```python
from build123d import *

# Parameters (mm, degrees)
F1_W     = 30
F1_H     = 30
F1_W_2   = 27
F1_H_2   = 27
F3_R     = 5
F5_DEPTH = 40
F4_R     = 5
F6_DEPTH = 40


with BuildPart() as f2:
    # F2: sweep along a path in F0
    with BuildLine(Plane.YZ) as f2_path:
        Line((0, 0), (0, 750))
        ThreePointArc((0, 750), (29.2893218813, 820.7106781187), (100, 850))
        Line((100, 850), (368.5786437627, 850))
        ThreePointArc((368.5786437627, 850), (406.8469869992, 842.3879532511), (439.2893218813, 820.7106781187))
        Line((439.2893218813, 820.7106781187), (470.7106781187, 789.2893218813))
        ThreePointArc((470.7106781187, 789.2893218813), (503.1530130008, 767.6120467489), (541.4213562373, 760))
        Line((541.4213562373, 760), (820, 760))
        ThreePointArc((820, 760), (890.7106781187, 730.7106781187), (920, 660))
        Line((920, 660), (920, 0))
    # F1 (on Top) → F2 (sweep)
    with BuildSketch(Plane.XY):
        Rectangle(F1_W, F1_H)
        Rectangle(F1_W_2, F1_H_2, mode=Mode.SUBTRACT)
    sweep(path=f2_path.line)

    # F3 (on face) → F5 (cut)
    with BuildSketch(Plane.XY.offset(865)):
        with Locations((0, 130)):
            Circle(F3_R)
        with Locations((0, 338.5786437627)):
            Circle(F3_R)
    extrude(amount=-F5_DEPTH, mode=Mode.SUBTRACT)

    # F4 (on face) → F6 (cut)
    with BuildSketch(Plane.XY.offset(775)):
        with Locations((0, 571.4213562373)):
            Circle(F4_R)
        with Locations((0, 790)):
            Circle(F4_R)
    extrude(amount=-F6_DEPTH, mode=Mode.SUBTRACT)


solid = f2.part
```
Geometry: final body of the model. Coordinates: model frame, mm. A direction names the side the tool comes from. Coordinates: 2 decimals unless noted, no trailing zeros. Order: outer loops, then holes, each group sorted by start corner. A loop starts at its lowest first (then second) coordinate and runs counter-clockwise, first axis right, second up. Notation, with made-up numbers: (-1, 42.25) -> (28, 42.25) arc R32 ccw to (28, 81.25) -> close; hole circle Ø11 at (83, -14.75). An arc over 180 degrees is marked (long way). Write each question's results on one line, items separated by ' | '. Start each with the question number.
1) Cut plane C-C, the plane x = 0. State how many separate pieces and enclosed holes the cut face has, and give its area (3 significant figures).
2) First-contact query: pin 1 (15 mm diameter, centred on x = 5, y = 621, fed in from -Z); pin 2 (8 mm diameter, centred on x = 0, y = 790, fed in from -Z); pin 3 (15 mm diameter, centred on x = 1, y = 213.5, fed in from -Z); pin 4 (8 mm diameter, centred on x = -3.5, y = 440.5, fed in from +Z). Flat tips, straight axial feed; report the tip coordinate or a pass-through.
3) Cut plane B-B, the plane y = 146.5. Output: boundary loops of the cut face in (x, z).
4) Set-up query: faces 4 (the flat face through (0, 683, 775)), 5 (the cylindrical face through (0.19, 497.41, 755.38)), 6 (the cylindrical face through (-0.2, 39.2, 809.4)). Return all of +Z, -Z, +X, -X, +Y, -Y with unobstructed straight access to the full face (end or side cutting, diameter ignored); none if empty.
5) Material intervals for line 1 along Y through (x, z) = (0.5, 569.5); line 2 along Z through (x, y) = (12, 805); line 3 along X through (y, z) = (790, 774), sorted ascending.
6) Cut plane A-A, the plane z = 561.5. Output: boundary loops of the cut face in (x, y), and give its area (3 significant figures).
7) Cut plane D-D, the plane z = 734. Output: boundary loops of the cut face in (x, y), and give its area (3 significant figures).
8) Mould query, pull axis X, two halves, no side actions, for faces 1 (the flat face through (15, 528, 755)), 2 (the cylindrical face through (0.189, 401.241, 830.096)), 3 (the flat face through (14, 921, 0)). Classes: released by +X, released by -X, zero draft, split by the parting line, or undercut.
Checks:
1) separate pieces: 10 | enclosed holes: 0 | area: 7,300 mm^2
2) pin 1: z = 745 | pin 2: through | pin 3: z = 835 | pin 4: z = 842.8
3) outline: (-15, 835) -> (15, 835) -> (15, 865) -> (-15, 865) -> close; hole (-13.5, 836.5) -> (13.5, 836.5) -> (13.5, 863.5) -> (-13.5, 863.5) -> close
4) face 4: +Z, +X, -X, +Y | face 5: none | face 6: -Z, +X, -X
5) line 1: -15 to -13.5, 13.5 to 15, 905 to 906.5, 933.5 to 935 | line 2: 745 to 746.5, 773.5 to 775 | line 3: -15 to -5, 5 to 15
6) outline: (-15, -15) -> (15, -15) -> (15, 15) -> (-15, 15) -> close; (-15, 905) -> (15, 905) -> (15, 935) -> (-15, 935) -> close; hole (-13.5, -13.5) -> (13.5, -13.5) -> (13.5, 13.5) -> (-13.5, 13.5) -> close; hole (-13.5, 906.5) -> (13.5, 906.5) -> (13.5, 933.5) -> (-13.5, 933.5) -> close | area: 342 mm^2
7) outline: (-15, -15) -> (15, -15) -> (15, 15) -> (-15, 15) -> close; (-15, 861.82) -> (15, 861.82) -> (15, 908.03) -> (-15, 908.03) -> close; hole (-13.5, -13.5) -> (13.5, -13.5) -> (13.5, 13.5) -> (-13.5, 13.5) -> close; hole (-13.5, 864.79) -> (13.5, 864.79) -> (13.5, 906.06) -> (-13.5, 906.06) -> close | area: 443 mm^2
8) face 1: released by +X | face 2: undercut | face 3: zero draft
